```python
from build123d import *

# Parameters (mm, degrees)
SKETCH1_W           = 82
SKETCH1_H           = 122
BOSS_EXTRUDE1_DEPTH = 23
SKETCH2_W           = 76
SKETCH2_H           = 116
CUT_EXTRUDE1_DEPTH  = 21
SKETCH6_W           = 78
SKETCH6_H           = 118
CUT_EXTRUDE3_DEPTH  = 2


with BuildPart() as part:
    # Sketch1 → Boss-Extrude1 (new body)
    with BuildSketch(Plane.XY):
        Rectangle(SKETCH1_W, SKETCH1_H)
    extrude(amount=-BOSS_EXTRUDE1_DEPTH)

    # Sketch2 → Cut-Extrude1 (cut)
    with BuildSketch(Plane(origin=(0, 0, -23), x_dir=(-1, 0, 0), z_dir=(0, 0, -1))):
        Rectangle(SKETCH2_W, SKETCH2_H)
    extrude(amount=-CUT_EXTRUDE1_DEPTH, mode=Mode.SUBTRACT)

    # Sketch6 → Cut-Extrude3 (cut)
    with BuildSketch(Plane(origin=(0, 0, -23), x_dir=(-1, 0, 0), z_dir=(0, 0, -1))):
        Rectangle(SKETCH6_W, SKETCH6_H)
    extrude(amount=-CUT_EXTRUDE3_DEPTH, mode=Mode.SUBTRACT)


solid = part.part
```
The model under review builds one solid part; all positions refer to its coordinate system, in mm. A direction names the side the tool comes from. Round coordinates to 2 decimals unless told otherwise and drop trailing zeros. Loops run counter-clockwise (first coordinate to the right, second up) from the corner with the lowest first, then second, coordinate; pieces in that order, holes last. Notation, with made-up numbers: (89, 17) - (97, 17) arc R25 cw to (97, 29) - close; hole circle Ø10 at (-32, 87). An arc over 180 degrees is marked (long way). Use a Markdown table: item, result. Add a question column.
Q1. Add section B-B (y = -29). State the section outline as (x, z) points.
Q2. Insertion check: pin 1 Ø4 at (x, y) = (8, -10.5) entering from +Z; pin 2 Ø23.5 at (x, y) = (14.5, -14.5) entering from -Z. Each pin has a flat end and moves straight along its axis. Give the tip position at first contact, or say it passes through.
Q3. For probe 1 along X at (y, z) = (-8, -10); probe 2 along Y at (x, z) = (-11.5, -22); probe 3 along Y at (x, z) = (11.5, -14.25), list the stretches that pass through material, from the lowest coordinate up.
Q4. Machinability: for faces 1 (the face through (41, -1, -11)), 2 (the face through (-38, -1, -12)), which of the approach directions +Z, -Z, +X, -X, +Y, -Y give a long, thin tool a straight path to every point of the face, cutting with its end or side? Answer none if there is none.
Q5. Add section C-C (z = -14). State the section outline as (x, y) points, plus the area to 3 significant figures.
Q6. Add section A-A (x = -4). State the section outline as (y, z) points.
Worked answers:
| question | item | result |
|---|---|---|
| 1 | outline | (-41, -23) - (-39, -23) - (-39, -21) - (-38, -21) - (-38, -2) - (38, -2) - (38, -21) - (39, -21) - (39, -23) - (41, -23) - (41, 0) - (-41, 0) - close |
| 2 | pin 1 | z = 0 |
| 2 | pin 2 | z = -2 |
| 3 | probe 1 | -41 to -38, 38 to 41 |
| 3 | probe 2 | -61 to -59, 59 to 61 |
| 3 | probe 3 | -61 to -58, 58 to 61 |
| 4 | face 1 | +Z, -Z, +X, +Y, -Y |
| 4 | face 2 | -Z |
| 5 | outline | (-41, -61) - (41, -61) - (41, 61) - (-41, 61) - close; hole (-38, -58) - (38, -58) - (38, 58) - (-38, 58) - close |
| 5 | area | 1,190 mm² |
| 6 | outline | (-61, -23) - (-59, -23) - (-59, -21) - (-58, -21) - (-58, -2) - (58, -2) - (58, -21) - (59, -21) - (59, -23) - (61, -23) - (61, 0) - (-61, 0) - close |
